The drawing under review shows one solid part. Ordinate dimensions are in mm from its lowest x, y, z. Coordinates: 2 decimals unless noted, no trailing zeros. Write each loop counter-clockwise with the first axis right and the second up, starting at its lowest first coordinate (ties: lowest second). Pieces come first, ordered by that corner, then holes.
Q1. To check wall thickness, follow probe 1 along Z at (x, y) = (37, 25); probe 2 along Y at (x, z) = (22, 18.25) (1 decimal); probe 3 along Y at (x, z) = (41, 3.75) (1 decimal). State the ranges of each line that lie inside material, in increasing order.
Q2. The part is to be moulded in two halves that separate along Y. For the marked faces 1, 2 and 3, say which applies: +Y half, -Y half, draft (parallel to the pull), parting line (faces both ways), or undercut.
Q3. Add section A-A, the plane x = 25.4. Give the boundary of the cut face in (y, z).
Q4. Clearance check with flat-ended pins moving along their axes: pin 1 Ø10 at (x, z) = (20, 7.5) entering from -Y; pin 2 Ø1.5 at (x, z) = (45, 13) entering from +Y (1 decimal); pin 3 Ø2 at (x, z) = (40, 2) entering from -Y; pin 4 Ø2 at (x, y) = (32, 7) entering from -Z. State where each tip first meets the part, or that it passes through.
Q5. Add section B-B, the plane z = 6.75. Give the boundary of the cut face in (x, y).
Q6. Add section C-C, the plane z = 12. Give the boundary of the cut face in (x, y).
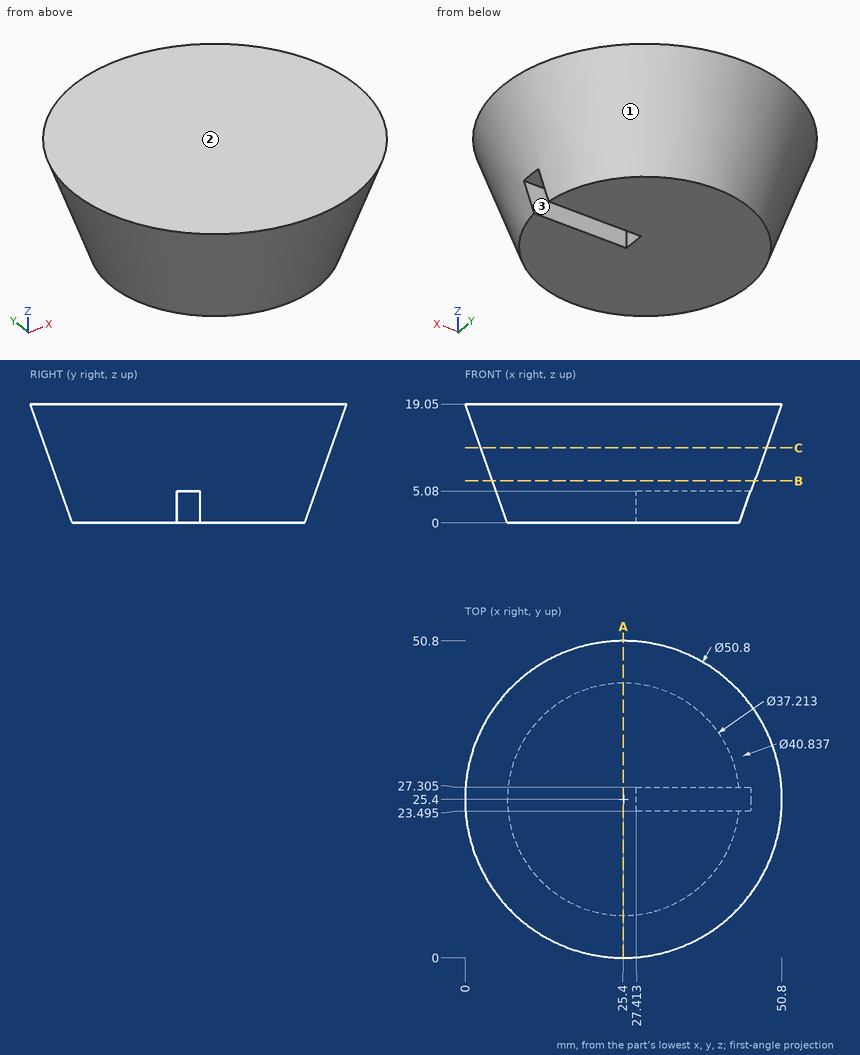
Here are the results:
1. probe 1: z = 5.08 to 19.05
1. probe 2: y = 0.5 to 50.3
1. probe 3: y = 13 to 23.5, 27.3 to 37.8
2. face 1: parting line
2. face 2: draft
2. face 3: undercut
3. outline: (0, 19.05) - (6.79, 0) - (44.01, 0) - (50.8, 19.05) - close
4. pin 1: stops at y = 2.74
4. pin 2: stops at y = 39.1
4. pin 3: stops at y = 11.56
4. pin 4: stops at z = 0
5. outline: circle Ø42.03 at (25.4, 25.4)
6. outline: circle Ø45.77 at (25.4, 25.4)
